For this review, take the finished solid that the model builds, in its own axes (mm). Coordinates: 2 decimals unless noted, no trailing zeros. Loops run counter-clockwise (first coordinate to the right, second up) from the corner with the lowest first, then second, coordinate; pieces in that order, holes last. Notation, with made-up numbers: (-29.75, -18) - (-13.75, -18) arc R19 ccw to (-13.75, 8) - close; hole circle Ø5 at (-27, 8.25). An arc over 180 degrees is marked (long way). Use one line per item in the form item = value. Start each with the question number.
1. Add section A-A on z = -9. Give the boundary of the cut face in (x, y).
2. Add section C-C on y = 0.7. Count the separate pieces of the cut face and the enclosed holes in it, and give its area (3 significant figures).
3. Add section D-D on z = 0. Give the boundary of the cut face in (x, y).
4. Draft analysis for pull direction X (two halves, no side actions). For faces 1 (the face through (0, 2, 0)), 2 (the face through (-8.93, 0.99, 20.09)), state which applies: +X half, -X half, draft (parallel to the pull), parting line (faces both ways), or undercut.
5. Add section B-B on y = 3.2. Give the boundary of the cut face in (x, z).
6. For pin 1 Ø5 at (x, z) = (-1, 18.5) entering from +Y; pin 2 Ø2 at (x, y) = (-14.5, 0.5) entering from +Z; pin 3 Ø2 at (y, z) = (2.5, -14.5) entering from -X, all flat-tipped, find the tip position at first contact; note any pin that passes through.
7. To check wall thickness, follow probe 1 along Y at (x, z) = (-4, 0.5); probe 2 along Z at (x, y) = (13.5, 1.1); probe 3 along X at (y, z) = (1.75, 5). State the ranges of each line that lie inside material, in increasing order.
```python
from build123d import *

# Parameters (mm, degrees)
SKETCH1_R           = 25
BOSS_EXTRUDE1_DEPTH = 2
SKETCH2_R           = 1.05
SKETCH2_R_2         = 0.79375
CUT_EXTRUDE1_DEPTH  = 36.411862419
SKETCH4_R           = 2.05
CUT_EXTRUDE3_DEPTH  = 36.411862419
BOSS_EXTRUDE2_START = 4
SKETCH7_R           = 0.79375
SKETCH7_R_2         = 0.77375
BOSS_EXTRUDE2_DEPTH = 4


with BuildPart() as part:
    # Sketch1 → Boss-Extrude1 (new body)
    with BuildSketch(Plane(origin=(0, 0, 0), x_dir=(1, 0, 0), z_dir=(0, 1, 0))):
        with Locations(Location((0, 0, 0), (0, 0, 270))):
            Circle(SKETCH1_R)
    extrude(amount=BOSS_EXTRUDE1_DEPTH)

    # Sketch2 → Cut-Extrude1 (cut, through all)
    with BuildSketch(Plane(origin=(0, 2, 0), x_dir=(1, 0, 0), z_dir=(0, 1, 0))):
        with Locations(Location((-2.066368974, 7.209723938, 0), (0, 0, 270))):
            Circle(SKETCH2_R)
        with Locations(Location((7.209723938, 2.066368974, 0), (0, 0, 270))):
            Circle(SKETCH2_R)
        with Locations(Location((2.066368974, -7.209723938, 0), (0, 0, 270))):
            Circle(SKETCH2_R)
        with Locations(Location((-7.209723938, -2.066368974, 0), (0, 0, 270))):
            Circle(SKETCH2_R)
        with Locations(Location((-3.636901173, -6.559188201, 0), (0, 0, 270))):
            Circle(SKETCH2_R_2)
        with Locations(Location((-6.559188201, 3.636901173, 0), (0, 0, 270))):
            Circle(SKETCH2_R_2)
        with Locations(Location((3.636901173, 6.559188201, 0), (0, 0, 270))):
            Circle(SKETCH2_R_2)
        with Locations(Location((6.559188201, -3.636901173, 0), (0, 0, 270))):
            Circle(SKETCH2_R_2)
    extrude(amount=-CUT_EXTRUDE1_DEPTH, mode=Mode.SUBTRACT)

    # Sketch4 → Cut-Extrude3 (cut, through all)
    with BuildSketch(Plane.XZ):
        with Locations(Location((-18.488747294, 7.626678405, 0), (0, 0, 270))):
            Circle(SKETCH4_R)
        with Locations(Location((-7.680642569, 18.466394605, 0), (0, 0, 270))):
            Circle(SKETCH4_R)
        with Locations(Location((7.626678405, 18.488747294, 0), (0, 0, 270))):
            Circle(SKETCH4_R)
        with Locations(Location((18.466394605, 7.680642569, 0), (0, 0, 270))):
            Circle(SKETCH4_R)
        with Locations(Location((18.488747294, -7.626678405, 0), (0, 0, 270))):
            Circle(SKETCH4_R)
        with Locations(Location((7.680642569, -18.466394605, 0), (0, 0, 270))):
            Circle(SKETCH4_R)
        with Locations(Location((-7.626678405, -18.488747294, 0), (0, 0, 270))):
            Circle(SKETCH4_R)
        with Locations(Location((-18.466394605, -7.680642569, 0), (0, 0, 270))):
            Circle(SKETCH4_R)
    extrude(amount=-CUT_EXTRUDE3_DEPTH, mode=Mode.SUBTRACT)

    # Sketch7 → Boss-Extrude2 (add)
    # profile 1 of 4: a face of its own
    with BuildSketch(Plane(origin=(0, 0, 0), x_dir=(1, 0, 0), z_dir=(0, 1, 0)).offset(BOSS_EXTRUDE2_START)):
        with Locations(Location((-3.636901173, -6.559188201, 0), (0, 0, 270))):
            Circle(SKETCH7_R)
        with Locations(Location((-3.636901173, -6.559188201, 0), (0, 0, 270))):
            Circle(SKETCH7_R_2, mode=Mode.SUBTRACT)
    # profile 2 of 4: a face of its own
    with BuildSketch(Plane(origin=(0, 0, 0), x_dir=(1, 0, 0), z_dir=(0, 1, 0)).offset(BOSS_EXTRUDE2_START)):
        with Locations(Location((6.559188201, -3.636901173, 0), (0, 0, 270))):
            Circle(SKETCH7_R)
        with Locations(Location((6.559188201, -3.636901173, 0), (0, 0, 270))):
            Circle(SKETCH7_R_2, mode=Mode.SUBTRACT)
    # profile 3 of 4: a face of its own
    with BuildSketch(Plane(origin=(0, 0, 0), x_dir=(1, 0, 0), z_dir=(0, 1, 0)).offset(BOSS_EXTRUDE2_START)):
        with Locations(Location((-6.559188201, 3.636901173, 0), (0, 0, 270))):
            Circle(SKETCH7_R)
        with Locations(Location((-6.559188201, 3.636901173, 0), (0, 0, 270))):
            Circle(SKETCH7_R_2, mode=Mode.SUBTRACT)
    # profile 4 of 4: a face of its own
    with BuildSketch(Plane(origin=(0, 0, 0), x_dir=(1, 0, 0), z_dir=(0, 1, 0)).offset(BOSS_EXTRUDE2_START)):
        with Locations(Location((3.636901173, 6.559188201, 0), (0, 0, 270))):
            Circle(SKETCH7_R)
        with Locations(Location((3.636901173, 6.559188201, 0), (0, 0, 270))):
            Circle(SKETCH7_R_2, mode=Mode.SUBTRACT)
    extrude(amount=-BOSS_EXTRUDE2_DEPTH)


solid = part.part
```
Conclusion:
q1.outline = (-23.32, 0) - (-20.04, 0) - (-20.04, 2) - (-23.32, 2) - close; (-16.9, 0) - (16.97, 0) - (16.97, 2) - (-16.9, 2) - close; (20.01, 0) - (23.32, 0) - (23.32, 2) - (20.01, 2) - close
q2.separate_pieces = 1
q2.enclosed_holes = 16
q2.area = 1,840 mm^2
q3.outline = (-25, 0) - (25, 0) - (25, 2) - (-25, 2) - close
q4.face_1 = draft
q4.face_2 = undercut
q5.outline = circle Ø1.59 at (-6.56, -3.64); circle Ø1.59 at (-3.64, 6.56); circle Ø1.59 at (3.64, -6.56); circle Ø1.59 at (6.56, 3.64); hole circle Ø1.55 at (-6.56, -3.64); hole circle Ø1.55 at (-3.64, 6.56); hole circle Ø1.55 at (3.64, -6.56); hole circle Ø1.55 at (6.56, 3.64)
q6.pin_1 = 2
q6.pin_2 = 21.04
q6.pin_3 = -20.96
q7.probe_1 = 0 to 2
q7.probe_2 = -21.04 to 21.04
q7.probe_3 = -24.49 to 24.49
